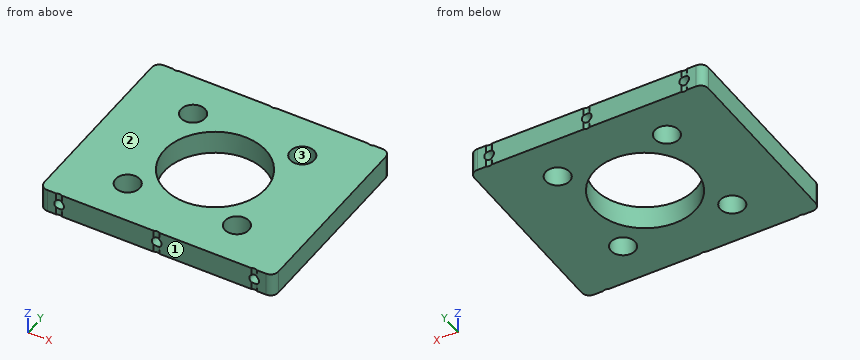
Autodesk Inventor part; units mm, degrees
ref_plane "YZ Plane" through (0, 0, 0) normal (1, 0, 0) x (0, 1, 0)
ref_plane "XZ Plane" through (0, 0, 0) normal (0, 1, 0) x (-1, 0, 0)
ref_plane "XY Plane" through (0, 0, 0) normal (0, 0, 1) x (1, 0, 0)
sketch "スケッチ1" plane through (0, 0, 0) normal (0, 0, 1) x (1, 0, 0)
  circle A0 centre (0, 0) radius 13
  circle A1 centre (-14, 14) radius 3.1
  circle A2 centre (14, 14) radius 3.1
  circle A3 centre (-14, -14) radius 3.1
  circle A4 centre (14, -14) radius 3.1
  line L0 (20, 20) -> (-20, 20) construction
  line L1 (-20, 20) -> (-20, -20) construction
  line L2 (-20, -20) -> (20, -20) construction
  line L3 (20, -20) -> (20, 20) construction
  line L4 (20, 20) -> (-20, -20) construction
  line L5 (-20, 20) -> (20, -20) construction
  line L6 (30, 25) -> (25.7483, 25)
  line L7 (-30, 25) -> (-30, -25)
  line L8 (-30, -25) -> (-25.7483, -25)
  line L9 (30, -25) -> (30, 25)
  line L10 (30, 25) -> (-30, -25) construction
  line L11 (-30, 25) -> (30, -25) construction
  arc A5 (-0.7483, 25) -> (0.7483, 25) centre (0, 26.3) ccw
  arc A6 (-25.7483, 25) -> (-24.2517, 25) centre (-25, 26.3) ccw
  arc A7 (24.2517, 25) -> (25.7483, 25) centre (25, 26.3) ccw
  arc A8 (-24.2517, -25) -> (-25.7483, -25) centre (-25, -26.3) ccw
  arc A9 (0.7483, -25) -> (-0.7483, -25) centre (0, -26.3) ccw
  arc A10 (25.7483, -25) -> (24.2517, -25) centre (25, -26.3) ccw
  arc A11 (-24.2517, 25) -> (-25.7483, 25) centre (-25, 26.3) ccw construction
  arc A12 (0.7483, 25) -> (-0.7483, 25) centre (0, 26.3) ccw construction
  arc A13 (25.7483, 25) -> (24.2517, 25) centre (25, 26.3) ccw construction
  arc A14 (-25.7483, -25) -> (-24.2517, -25) centre (-25, -26.3) ccw construction
  arc A15 (-0.7483, -25) -> (0.7483, -25) centre (0, -26.3) ccw construction
  arc A16 (24.2517, -25) -> (25.7483, -25) centre (25, -26.3) ccw construction
  line L12 (-24.2517, 25) -> (-25.7483, 25) construction
  line L13 (-25.7483, 25) -> (-30, 25)
  line L14 (-0.7483, 25) -> (-24.2517, 25)
  line L15 (0.7483, 25) -> (-0.7483, 25) construction
  line L16 (25.7483, 25) -> (24.2517, 25) construction
  line L17 (24.2517, 25) -> (0.7483, 25)
  line L18 (-24.2517, -25) -> (-0.7483, -25)
  line L19 (-25.7483, -25) -> (-24.2517, -25) construction
  line L20 (0.7483, -25) -> (24.2517, -25)
  line L21 (-0.7483, -25) -> (0.7483, -25) construction
  line L22 (25.7483, -25) -> (30, -25)
  line L23 (24.2517, -25) -> (25.7483, -25) construction
  dimension "d0" = 26
  dimension "d1" = 6.2
  dimension "d2" = 6.2
  dimension "d3" = 6.2
  dimension "d4" = 6.2
  dimension "d5" = 28
  dimension "d6" = 28
  dimension "d7" = 14
  dimension "d8" = 14
  dimension "d9" = 40
  dimension "d10" = 40
  dimension "d11" = 10
  dimension "d12" = 5
  dimension "d13" = 3
  dimension "d14" = 3
  dimension "d15" = 3
  dimension "d16" = 3
  dimension "d17" = 3
  dimension "d18" = 3
  dimension "d19" = 1.3
  dimension "d20" = 1.3
  dimension "d21" = 25
  dimension "d22" = 25
extrude "押し出し1" add sketch "スケッチ1" along normal blind 6
sketch "スケッチ2" plane through (-24.2517, 25, 0) normal (0, 1, 0) x (1, 0, 0)
  circle A0 centre (-0.7483, -3) radius 1.25
  circle A1 centre (24.2517, -3) radius 1.25
  circle A2 centre (49.2517, -3) radius 1.25
  point P0 (24.2517, 0)
  dimension "d25" = 2.5
  dimension "d26" = 2.5
  dimension "d27" = 2.5
  dimension "d28" = 25
  dimension "d29" = 25
  dimension "d30" = 3
extrude "押し出し2" cut sketch "スケッチ2" against normal blind 6
sketch "スケッチ3" plane through (-24.2517, -25, 0) normal (0, -1, 0) x (1, 0, 0)
  circle A0 centre (24.2517, 3) radius 1.25
  circle A1 centre (-0.7483, 3) radius 1.25
  circle A2 centre (49.2517, 3) radius 1.25
  point P0 (24.2517, 0)
extrude "押し出し3" cut sketch "スケッチ3" against normal blind 6
fillet "フィレット1" radius 2 4 edges at (-30, 25, 3) (30, 25, 3) (30, -25, 3) (-30, -25, 3)
properties part number "ハンド_エアシリンダ固定具" material "ポリカーボネート、スモーク"
Read the model definition and answer for the solid it produces. Units are mm, in the model's axes. Face numbers are marked on the shaded views. Give positions to 0.01 mm unless a question says otherwise; leave off trailing zeros. Write each loop counter-clockwise with the first axis right and the second up, starting at its lowest first coordinate (ties: lowest second). Pieces come first, ordered by that corner, then holes. Notation, with made-up numbers: (-5.75, -31) - (21.25, -31) arc R27 ccw to (21.25, 0) - close; hole circle Ø10 at (-8.5, 9). An arc over 180 degrees is marked (long way). Use CSV: the item, a comma, the result in double quotes. Start each with the question number.
Item 1: Consider line 1 (Y direction, x = -14, z = 4.05); line 2 (X direction, y = -20.75, z = 3); line 3 (Z direction, x = 0, y = 22.25). Determine where each line is inside the solid, lowest interval first.
Item 2: The part is cut by section D-D, the plane x = 25. Give the vertices of the cut face in (y, z).
Item 3: The mould has two halves that part along Y. Classify the marked faces 1, 2 and 3: pulls with the +Y half, pulls with the -Y half, needs draft (parallel to the pull), parting line crosses it, or undercut.
Item 4: The part is cut by section B-B, the plane x = -2.5. Give the vertices of the cut face in (y, z), and give its area (3 significant figures).
Item 5: The part is cut by section A-A, the plane z = 1. Give the vertices of the cut face in (x, y).
Item 6: Flat-ended cylindrical pins translate along their axes: P1, Ø3, axis at x = 25, z = 3, coming from the -Y side; P2, Ø0.8, axis at x = 25, z = 2.5, coming from the +Y side; P3, Ø0.8, axis at x = 0, z = 2.5, coming from the -Y side. Find the tip coordinate at first contact, or state that the pin passes through.
Item 7: The part is cut by section C-C, the plane y = 0. Give the vertices of the cut face in (x, z).
Taken from the geometry:
1,line 1,"-25 to -17.1, -10.9 to 10.9, 17.1 to 25"
1,line 2,"-30 to -26.25, -23.75 to -1.25, 1.25 to 23.75, 26.25 to 30"
1,line 3,"0 to 1.75, 4.25 to 6"
2,outline,"(-24.8, 0) - (24.8, 0) - (24.8, 1.75) - (19, 1.75) - (19, 4.25) - (24.8, 4.25) - (24.8, 6) - (-24.8, 6) - (-24.8, 4.25) - (-19, 4.25) - (-19, 1.75) - (-24.8, 1.75) - close"
3,face 1,"pulls with the -Y half"
3,face 2,"needs draft"
3,face 3,"undercut"
4,outline,"(-25, 0) - (-12.76, 0) - (-12.76, 6) - (-25, 6) - close; (12.76, 0) - (25, 0) - (25, 6) - (12.76, 6) - close"
4,area,"147 mm2"
5,outline,"(-30, -23) arc R2 ccw to (-28, -25) - (-25.75, -25) arc R1.5 cw to (-24.25, -25) - (-0.75, -25) arc R1.5 cw to (0.75, -25) - (24.25, -25) arc R1.5 cw to (25.75, -25) - (28, -25) arc R2 ccw to (30, -23) - (30, 23) arc R2 ccw to (28, 25) - (25.75, 25) arc R1.5 cw to (24.25, 25) - (0.75, 25) arc R1.5 cw to (-0.75, 25) - (-24.25, 25) arc R1.5 cw to (-25.75, 25) - (-28, 25) arc R2 ccw to (-30, 23) - close; hole circle Ø6.2 at (-14, -14); hole circle Ø6.2 at (-14, 14); hole circle Ø26 at (0, 0); hole circle Ø6.2 at (14, -14); hole circle Ø6.2 at (14, 14)"
6,P1,"y = -25"
6,P2,"y = 19"
6,P3,"y = -19"
7,outline,"(-30, 0) - (-13, 0) - (-13, 6) - (-30, 6) - close; (13, 0) - (30, 0) - (30, 6) - (13, 6) - close"
